Answer from the drawing. Dimensions are ordinates in mm from the lowest x, y and z of the part. Coordinates: 2 decimals unless noted, no trailing zeros. Loops run counter-clockwise (first coordinate to the right, second up) from the corner with the lowest first, then second, coordinate; pieces in that order, holes last.
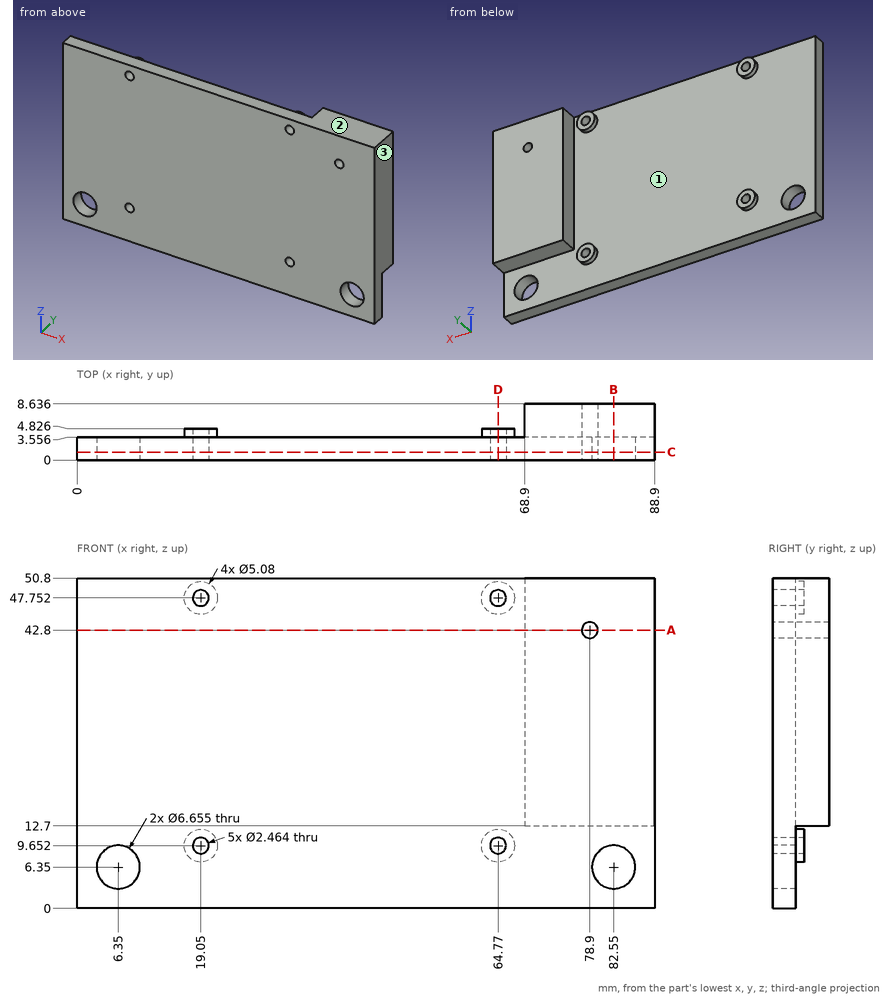
Item 1: Determine the mould class of the marked faces 1, 2 and 3 for opening direction X: released by +X, released by -X, zero draft, split by the parting line, or undercut.
Numbers:
face 1: undercut
face 2: zero draft
face 3: released by +X
Item 2: A cutting plane is placed at B-B on x = 82.55. Determine the outline of the cut face in (y, z).
Numbers:
outline: (0, 0) - (3.56, 0) - (3.56, 3.02) - (0, 3.02) - close; (0, 9.68) - (3.56, 9.68) - (3.56, 12.7) - (8.64, 12.7) - (8.64, 50.8) - (0, 50.8) - close
Item 3: Find the intervals of material crossed by line 1 along X through (y, z) = (1.95, 6.35); line 2 along X through (y, z) = (3.25, 3.5); line 3 along X through (y, z) = (2, 9) (1 decimal), in increasing order.
Numbers:
line 1: x = 0 to 3.02, 9.68 to 79.22, 85.88 to 88.9
line 2: x = 0 to 4.63, 8.07 to 80.83, 84.27 to 88.9
line 3: x = 0 to 4.3, 8.4 to 18, 20.1 to 63.7, 65.8 to 80.5, 84.6 to 88.9
Item 4: Given pin 1 (7.5 mm diameter, centred on x = 82.55, z = 6.35, fed in from +Y); pin 2 (12 mm diameter, centred on x = 9, z = 18.5, fed in from -Y); pin 3 (4 mm diameter, centred on x = 19.5, z = 48, fed in from +Y); pin 4 (1.5 mm diameter, centred on y = 5, z = 35.5, fed in from -X), each flat-ended and moving along its own axis, determine where each tip first touches the part or whether it passes through.
Numbers:
pin 1: stops at y = 3.56
pin 2: stops at y = 0
pin 3: stops at y = 4.83
pin 4: stops at x = 68.9
Item 5: A cutting plane is placed at A-A on z = 42.8. Determine the outline of the cut face in (x, y).
Numbers:
outline: (0, 0) - (77.67, 0) - (77.67, 8.64) - (68.9, 8.64) - (68.9, 3.56) - (0, 3.56) - close; (80.13, 0) - (88.9, 0) - (88.9, 8.64) - (80.13, 8.64) - close
Item 6: A cutting plane is placed at C-C on y = 1.25. Give the number of separate pieces and of enclosed holes in the cut face, then the cut area to 3 significant figures.
Numbers:
separate pieces: 1
enclosed holes: 7
area: 4,420 mm2
Item 7: A cutting plane is placed at D-D on x = 64.77. Determine the outline of the cut face in (y, z), then the cut area to 3 significant figures.
Numbers:
outline: (0, 0) - (3.56, 0) - (3.56, 7.11) - (4.83, 7.11) - (4.83, 8.42) - (0, 8.42) - close; (0, 10.88) - (4.83, 10.88) - (4.83, 12.19) - (3.56, 12.19) - (3.56, 45.21) - (4.83, 45.21) - (4.83, 46.52) - (0, 46.52) - close; (0, 48.98) - (4.83, 48.98) - (4.83, 50.29) - (3.56, 50.29) - (3.56, 50.8) - (0, 50.8) - close
area: 170 mm2
